Drawing for the job (mm, zero at the part's lowest x, y, z). A direction names the side the tool comes from. Coordinates: 2 decimals unless noted, no trailing zeros. Write each loop counter-clockwise with the first axis right and the second up, starting at its lowest first coordinate (ties: lowest second). Pieces come first, ordered by that corner, then holes. Notation, with made-up numbers: (2.5, -38.5) -> (33.5, -38.5) arc R22 cw to (33.5, -25.5) -> close; hole circle Ø10 at (-9, 8). An arc over 180 degrees is marked (long way). Write item = value, one per line. Start each with the question number.
Q1. Tool access for the marked faces 4 and 5: list every direction of +Z, -Z, +X, -X, +Y, -Y with a clear straight run to the whole face (end or side of a thin tool).
Q2. Pull direction X, two halves, no side cores. Call the marked faces 1, 2 and 3: released by +X, released by -X, zero draft, split by the parting line, or undercut.
Q3. Band-saw the part on B-B, the plane y = 88. List the corners of the cut face in (x, z) (1 decimal), plus the area to 3 significant figures.
Q4. Band-saw the part on C-C, the plane x = 84.5. List the corners of the cut face in (y, z) (1 decimal).
Q5. Band-saw the part on A-A, the plane z = 53. List the corners of the cut face in (x, y).
Q6. Pin check, flat tip, straight feed: P1, Ø3, axis at x = 84, y = 71.5, coming from the +Z side. Stop position of the tip, or through.
Q7. Probe line 1 (X direction, y = 29, z = 79.5); line 2 (Y direction, x = 76.5, z = 14); line 3 (Z direction, x = 46, y = 43). List the from-to ranges inside material, lowest first.
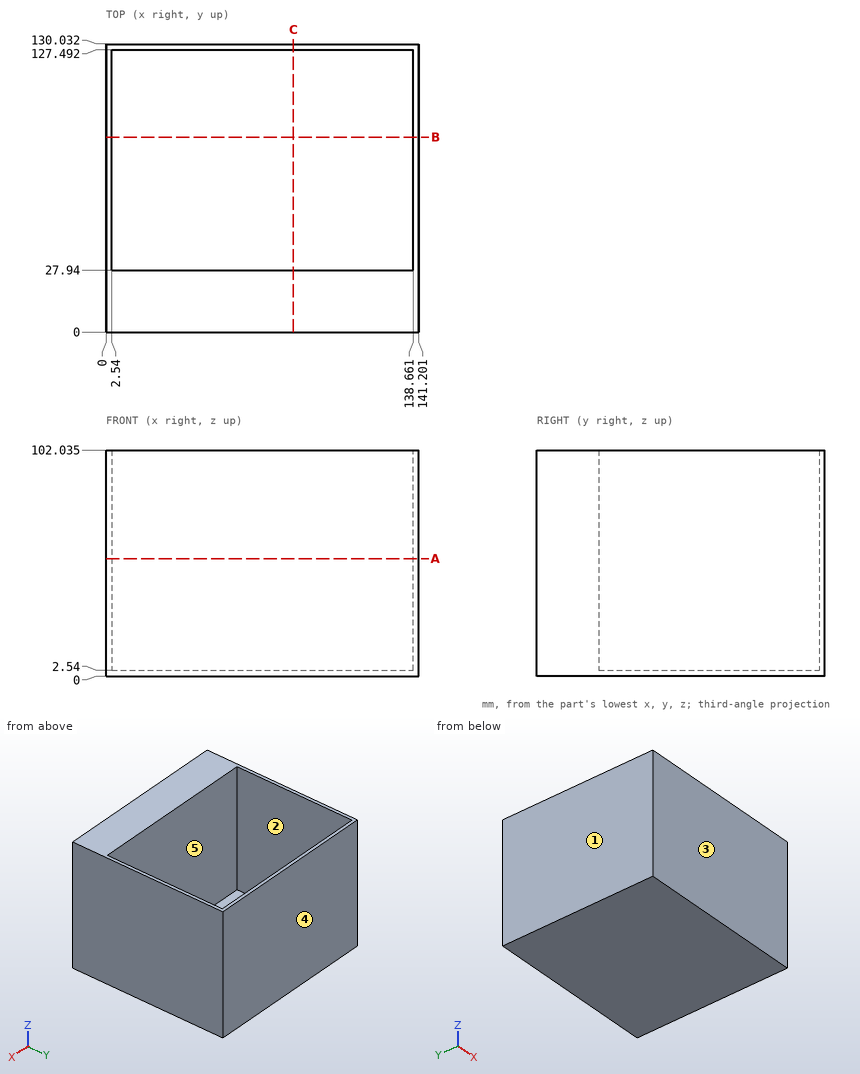
Ans:
q1.face_4 = +Z, -Z, +X, -X, +Y
q1.face_5 = +Z
q2.face_1 = released by -X
q2.face_2 = undercut
q2.face_3 = zero draft
q3.outline = (0, 0) -> (141.2, 0) -> (141.2, 102) -> (138.7, 102) -> (138.7, 2.5) -> (2.5, 2.5) -> (2.5, 102) -> (0, 102) -> close
q3.area = 864 mm2
q4.outline = (0, 0) -> (130, 0) -> (130, 102) -> (127.5, 102) -> (127.5, 2.5) -> (27.9, 2.5) -> (27.9, 102) -> (0, 102) -> close
q5.outline = (0, 0) -> (141.2, 0) -> (141.2, 130.03) -> (0, 130.03) -> close; hole (2.54, 27.94) -> (138.66, 27.94) -> (138.66, 127.49) -> (2.54, 127.49) -> close
q6.P1 = 2.54
q7.line_1 = 0 to 2.54, 138.66 to 141.2
q7.line_2 = 0 to 27.94, 127.49 to 130.03
q7.line_3 = 0 to 2.54
